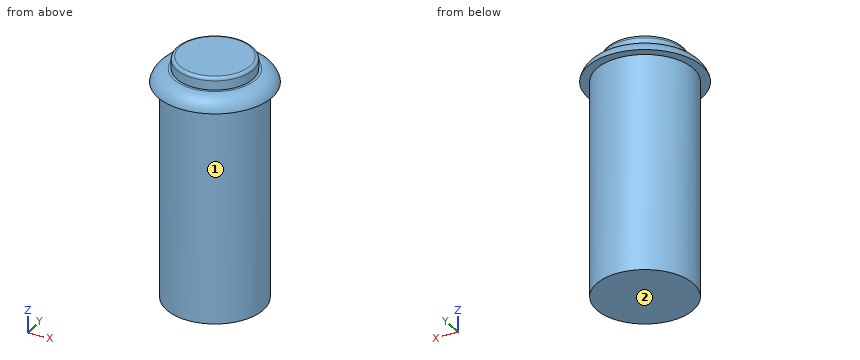
```python
from build123d import *

# Parameters (mm, degrees)
F0_R     = 16.51
F0_R_2   = 11.049
F1_DEPTH = 3.81
F2_DEPTH = 7.366
F4_R     = 0.889
F5_R     = 13.97
F5_R_2   = 11.049
F6_DEPTH = 62.23


# Not quite as in the source:
# - a fillet or chamfer that OpenCascade refuses, or shapes differently, is made with other operations: its cross-section is extruded or revolved along the edge and cut away or added


with BuildPart() as f1:
    # F0 (on Top) → F1 (new body)
    with BuildSketch(Plane.XY):
        Circle(F0_R)
        Circle(F0_R_2, mode=Mode.SUBTRACT)
    extrude(amount=F1_DEPTH)

    # F0 (on Top) → F2 (join)
    with BuildSketch(Plane.XY):
        Circle(F0_R_2)
    extrude(amount=F2_DEPTH)

    # F3: fillet of radius 4.826 on 1 edges, made by hand

    # F3_s1 → F3_t2 (revolve, cut)
    with BuildSketch(Plane.XZ):
        with BuildLine():
            ThreePointArc((16.51, 0), (14.8242428344, 2.7385633568), (11.7921593923, 3.81))
            Line((11.7921593923, 3.81), (16.51, 3.81))
            Line((16.51, 3.81), (16.51, 0))
        make_face()
    revolve(axis=Axis((0, 0, 3.81), (0, 0, 1)), mode=Mode.SUBTRACT)

    # F4
    f4_edges = [f1.edges().sort_by_distance(p)[0] for p in [
        (-11.049, 0, 7.366),
    ]]
    fillet(f4_edges, radius=F4_R)

    # F5 (on face) → F6 (join)
    with BuildSketch(Plane.XY):
        Circle(F5_R)
        Circle(F5_R_2, mode=Mode.SUBTRACT)
        Circle(F5_R_2)
    extrude(amount=-F6_DEPTH)


solid = f1.part
```
Work out the finished part from the listing and answer in its coordinate system (mm). Face numbers are marked on the shaded views. A direction names the side the tool comes from. Give positions to 0.01 mm unless a question says otherwise; leave off trailing zeros. Loops run counter-clockwise (first coordinate to the right, second up) from the corner with the lowest first, then second, coordinate; pieces in that order, holes last. Notation, with made-up numbers: (36, 38) - (90, 38) arc R26 ccw to (90, 66) - close; hole circle Ø10 at (54, 2.5). An arc over 180 degrees is marked (long way). Use CSV: the item, a comma, the result in double quotes. Start each with the question number.
(1) A tool of negligible diameter and unlimited length cuts with its end or side. For the marked faces 1 and 2, from which of +Z, -Z, +X, -X, +Y, -Y can it reach the whole face along a straight path? Write none if from no direction.
(2) Find section A-A, the plane y = 0. Determine the outline of the cut face in (x, z), plus the area to 3 significant figures.
(3) Each of these flat-tipped pins is pushed along its axis until it touches: pin 1 (8 mm diameter, centred on x = 10.5, y = -11.5, fed in from -Z); pin 2 (1 mm diameter, centred on x = 0, z = -34, fed in from +Y); pin 3 (3 mm diameter, centred on y = -2, z = -51.5, fed in from +X); pin 4 (1 mm diameter, centred on x = -7, z = -6, fed in from +Y). Where does it stop, or does it pass through?
(4) Find section C-C, the plane z = -40. Determine the outline of the cut face in (x, y), plus the area to 3 significant figures.
(5) Find the intervals of material crossed by L1, parallel to X at y = -0.5, z = -50; L2, parallel to Y at x = -12.5, z = -51.5; L3, parallel to X at y = 6, z = -40, in increasing order.
Results found:
1,face 1,"-Z"
1,face 2,"-Z, +X, -X, +Y, -Y"
2,outline,"(-16.51, 0) - (-13.97, 0) - (-13.97, -62.23) - (13.97, -62.23) - (13.97, 0) - (16.51, 0) arc R4.83 ccw to (11.79, 3.81) - (11.05, 3.81) - (11.05, 6.48) arc R0.89 ccw to (10.16, 7.37) - (-10.16, 7.37) arc R0.89 ccw to (-11.05, 6.48) - (-11.05, 3.81) - (-11.79, 3.81) arc R4.83 ccw to start"
2,area,"1,930 mm^2"
3,pin 1,"z = -62.23"
3,pin 2,"y = 13.97"
3,pin 3,"x = 13.96"
3,pin 4,"y = 12.37"
4,outline,"circle Ø27.94 at (0, 0)"
4,area,"613 mm^2"
5,L1,"-13.96 to 13.96"
5,L2,"-6.24 to 6.24"
5,L3,"-12.62 to 12.62"
